```python
from build123d import *

# Parameters (mm, degrees)
SKETCH_1_W             = 46
SKETCH_1_H             = 20
EXTRUDE_1_DEPTH        = 20
SKETCH_2_W             = 20
SKETCH_2_H             = 5.1
EXTRUDE_2_DEPTH        = 5
FILLET_1_R             = 2
FILLET_1_OF_MIRROR_1_R = 2
SKETCH_3_W             = 24
SKETCH_3_H             = 5
EXTRUDE_3_DEPTH        = 30
FILLET_2_R             = 18
FILLET_3_R             = 18


with BuildPart() as part:
    # 스케치1 → 보스-돌출1 (new body)
    with BuildSketch(Plane.XY):
        Rectangle(SKETCH_1_W, SKETCH_1_H)
    extrude(amount=EXTRUDE_1_DEPTH)

    # 스케치2 → 보스-돌출2 (add)
    with BuildSketch(Plane.ZY.offset(23)):
        with Locations((10, 0)):
            Rectangle(SKETCH_2_W, SKETCH_2_H)
    extrude_2 = extrude(amount=EXTRUDE_2_DEPTH)

    # 필렛1
    fillet_1_edges = [part.edges().sort_by_distance(p)[0] for p in [
        (-28, 2.55, 10),
        (-28, -2.55, 10),
    ]]
    fillet(fillet_1_edges, radius=FILLET_1_R)

    # 대칭 복사1: 보스-돌출2 across plane
    add(extrude_2.mirror(Plane(origin=(0, 0, 0), x_dir=(0, 0, 1), z_dir=(1, 0, 0))))

    # 필렛1 of 대칭 복사1
    fillet_1_of_mirror_1_edges = [part.edges().sort_by_distance(p)[0] for p in [
        (28, 2.55, 10),
        (28, -2.55, 10),
    ]]
    fillet(fillet_1_of_mirror_1_edges, radius=FILLET_1_OF_MIRROR_1_R)

    # 스케치3 → 보스-돌출3 (add)
    with BuildSketch(Plane(origin=(0, 0, 0), x_dir=(-1, 0, 0), z_dir=(0, 0, -1))):
        with Locations((0, -7.5)):
            Rectangle(SKETCH_3_W, SKETCH_3_H)
    extrude(amount=EXTRUDE_3_DEPTH)

    # 필렛2
    # the kernel refuses this fillet: 18 mm, written as the material it adds along each edge
    with BuildSketch(Plane(origin=(-12, -5, 0), x_dir=(0, 1, 0), z_dir=(1, 0, 0))) as fillet_2_piece_1:
        with BuildLine():
            CenterArc((18, -17.748239349), FILLET_2_R, 99.594068227, 80.405931773)
            Line((0, -17.748239349), (0, 0))
            Line((0, 0), (15, 0))
        make_face()
    extrude(amount=24)

    # 필렛3
    # the kernel refuses this fillet: 18 mm, written as the material it takes off along each edge
    with BuildSketch(Plane(origin=(-42.877791108, -5, -30), x_dir=(0, -1, 0), z_dir=(1, 0, 0))) as fillet_3_piece_1:
        with BuildLine():
            CenterArc((17.999451575, -12.45047223), FILLET_3_R, 136.235733455, 43.448005638)
            Line((-0.000274212, -12.35111644), (-1.800246791, -12.341180861))
            ThreePointArc((-1.800246791, -12.341180861), (-1.8, -12.251760651), (-1.8, 0))
            Line((-1.8, 0), (0, 1.8))
            ThreePointArc((0, 1.8), (2.5, 1.8), (3.700054842, 1.245047223))
            Line((3.700054842, 1.245047223), (5, 0))
        make_face()
    extrude(amount=85.755582217, mode=Mode.SUBTRACT)


solid = part.part
```
The model under review builds one solid part; all positions refer to its coordinate system, in mm. A direction names the side the tool comes from. Round coordinates to 2 decimals unless told otherwise and drop trailing zeros. Write each loop counter-clockwise with the first axis right and the second up, starting at its lowest first coordinate (ties: lowest second). Pieces come first, ordered by that corner, then holes. Notation, with made-up numbers: M 55,28.5 L 101,28.5 A22 cw 101,56.5 Z; hole C -0.5,-21.5 d4. An arc over 180 degrees is marked long. Use CSV: the item, a comma, the result in double quotes. Start each with the question number.
(1) For line 1 along Z through (x, y) = (21.5, -6.75); line 2 along X through (y, z) = (-8.5, -23); line 3 along X through (y, z) = (2.75, 9), list the stretches that pass through material, from the lowest coordinate up.
(2) Tool access review of faces 1 (the face through (-23, -6, 10)), 2 (the face through (-18, 0, 0)), 3 (the face through (23, -6, 10)), 4 (the face through (18, 0, 0)): name each direction out of +Z, -Z, +X, -X, +Y, -Y from which nothing blocks a thin tool from reaching the whole face with its end or side.
(3) We need section D-D, the plane x = 19. State the section outline as (y, z) points.
(4) We need section C-C, the plane y = 7.5. State the section outline as (x, z) points.
(5) We need section B-B, the plane x = 6. State the section outline as (y, z) points.
(6) Clearance check with flat-ended pins moving along their axes: P1, Ø1.5, axis at x = 25, z = 15, coming from the +Y side; P2, Ø3.5, axis at x = -25, z = 14, coming from the -Y side; P3, Ø0.9, axis at x = 24, z = 11, coming from the -Y side; P4, Ø12, axis at y = 7.5, z = -9, coming from the +X side. State where each tip first meets the part, or that it passes through.
(7) We need section A-A, the plane z = 3. State the section outline as (x, y) points.
(8) The part is to be moulded in two halves that separate along Y. For faces 5 (the face through (-23, 6, 10)), 6 (the face through (24, 2.55, 10)), 7 (the face through (27.4, -1.98, 10.14)), say which applies: +Y half, -Y half, draft (parallel to the pull), parting line (faces both ways), or undercut.
Findings:
1,line 1,"0 to 20"
1,line 2,"-12 to 12"
1,line 3,"-23 to 23"
2,face 1,"+Z, -Z, -X, -Y"
2,face 2,"-Z, -X, +Y, -Y"
2,face 3,"+Z, -Z, +X, -Y"
2,face 4,"-Z, +X, +Y, -Y"
3,outline,"M -10,0 L 10,0 L 10,20 L -10,20 Z"
4,outline,"M -23,0 L -12,0 L -12,-0.61 L 12,-0.61 L 12,0 L 23,0 L 23,20 L -23,20 Z"
5,outline,"M -10,-30 A18 ccw -5,-17.65 A18 cw 10,0 L 10,20 L -10,20 Z"
6,P1,"y = 2.55"
6,P2,"y = -2.55"
6,P3,"y = -2.55"
6,P4,"through"
7,outline,"M -28,-0.55 A2 ccw -26,-2.55 L -23,-2.55 L -23,-10 L 23,-10 L 23,-2.55 L 26,-2.55 A2 ccw 28,-0.55 L 28,0.55 A2 ccw 26,2.55 L 23,2.55 L 23,10 L -23,10 L -23,2.55 L -26,2.55 A2 ccw -28,0.55 Z"
8,face 5,"draft"
8,face 6,"+Y half"
8,face 7,"-Y half"
